Design review of the part built by this model. Coordinates are the model's own, in mm. Give positions to 0.01 mm unless a question says otherwise; leave off trailing zeros. Loops run counter-clockwise (first coordinate to the right, second up) from the corner with the lowest first, then second, coordinate; pieces in that order, holes last. Notation, with made-up numbers: M 80.5,-29.5 L 130.5,-29.5 A25 ccw 130.5,-6.5 Z; hole C -33,85 d8. An arc over 180 degrees is marked long. Use CSV: the item, a comma, the result in double quotes.
from build123d import *

# Parameters (mm, degrees)
F1_DEPTH = 3.175
F3_D     = 5.08


with BuildPart() as f1:
    # F0 (on Top) → F1 (new body)
    with BuildSketch(Plane.XY):
        with BuildLine():
            Line((25.4, 7.62), (0, 3.81))
            ThreePointArc((0, 3.81), (-3.81, 0), (0, -3.81))
            Line((0, -3.81), (25.4, -7.62))
            Line((25.4, -7.62), (30.48, -7.62))
            Line((30.48, -7.62), (30.48, 7.62))
            Line((30.48, 7.62), (25.4, 7.62))
        make_face()
    extrude(amount=F1_DEPTH)

    # F3 (through all)
    with Locations(Plane(origin=(0, 0, 0), x_dir=(1, 0, 0), z_dir=(0, 0, -1))):
        with Locations((0, 0)):
            Hole(F3_D / 2)


solid = f1.part
(1) The part is to be moulded in two halves that separate along Y. For faces 1 (the flat face through (12.52, -5.69, 1.57)), 2 (the cylindrical face through (0.33, -2.52, 1.61)), 3 (the flat face through (28, 7.62, 2)), 4 (the flat face through (17, 0, 3.175)), say which applies: released by +Y, released by -Y, zero draft, split by the parting line, or undercut.
A:
face 1,"released by -Y"
face 2,"undercut"
face 3,"released by +Y"
face 4,"zero draft"
(2) We need section D-D on y = 4.5. State the section outline as (x, z) points (3 decimals).
A:
outline,"M 4.6,0 L 30.48,0 L 30.48,3.175 L 4.6,3.175 Z"
(3) We need section A-A on y = 0. State the section outline as (x, z) points (3 decimals).
A:
outline,"M -3.81,0 L -2.54,0 L -2.54,3.175 L -3.81,3.175 Z; M 2.54,0 L 30.48,0 L 30.48,3.175 L 2.54,3.175 Z"
(4) We need section B-B on z = 1.7. State the section outline as (x, y) points, then the cut area to 3 significant figures.
A:
outline,"M 0,-3.81 L 25.4,-7.62 L 30.48,-7.62 L 30.48,7.62 L 25.4,7.62 L 0,3.81 A3.81 ccw Z; hole C 0,0 d5.08"
area,"370 mm²"
(5) Clearance check with a flat-ended pin moving along its axis: P1, Ø1, axis at x = 0.5, y = 5.5, coming from the -Z side. State where the tip first meets the part, or that it passes through.
A:
P1,"through"
(6) We need section C-C on x = 19. State the section outline as (y, z) points (3 decimals).
A:
outline,"M -6.66,0 L 6.66,0 L 6.66,3.175 L -6.66,3.175 Z"
(7) Wall thickness on line 1 along Y through (x, z) = (0, 2.1); line 2 along Y through (x, z) = (-1.5, 1); line 3 along X through (y, z) = (-1.75, 0.4): over which ranges is each line inside the solid? List them lowest first. Write a range as [from, to].
A:
line 1,"[-3.81, -2.54], [2.54, 3.81]"
line 2,"[-3.5, -2.05], [2.05, 3.5]"
line 3,"[-3.38, -1.84], [1.84, 30.48]"
